Source: CAD feature listing. Evaluate the final solid. Frame: model axes, mm. Face numbers are marked on the shaded views. A direction names the side the tool comes from. Round coordinates to 2 decimals unless told otherwise and drop trailing zeros. Loops run counter-clockwise (first coordinate to the right, second up) from the corner with the lowest first, then second, coordinate; pieces in that order, holes last. Notation, with made-up numbers: M 5,41.5 L 49,41.5 A21 ccw 49,77.5 Z; hole C 70,87.5 d9. An arc over 180 degrees is marked long. Answer as CSV lines item,"result". Start each with the question number.
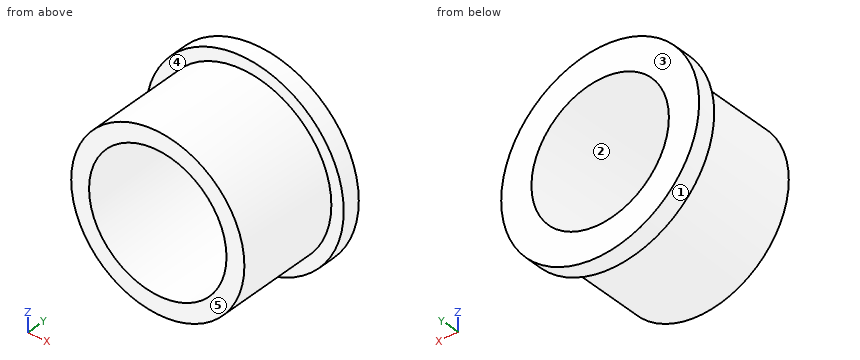
Autodesk Inventor part; units mm, degrees
ref_plane "YZ Plane" through (0, 0, 0) normal (1, 0, 0) x (0, 1, 0)
ref_plane "XZ Plane" through (0, 0, 0) normal (0, 1, 0) x (-1, 0, 0)
ref_plane "XY Plane" through (0, 0, 0) normal (0, 0, 1) x (1, 0, 0)
sketch "Sketch1" plane through (0, 0, 0) normal (0, 0, 1) x (1, 0, 0)
  line L0 (0, 0) -> (1.65, 0)
  line L1 (1.65, 0) -> (1.65, 3)
  line L2 (1.65, 3) -> (3.6, 3)
  line L3 (3.6, 3) -> (3.6, 3.65)
  line L4 (3.6, 3.65) -> (1.65, 3.65)
  line L5 (0, 0) -> (0, 3.65)
  line L6 (1.65, 3.65) -> (0, 3.65)
  dimension "d0" = 1.65
  dimension "d1" = 1.95
  dimension "d2" = 3
  dimension "d3" = 0.65
revolve "Revolution1" add sketch "Sketch1" angle 360 about axis through (0, 0, 0) along (0, 1, 0)
sketch "Sketch2" plane through (0, 0, 0) normal (1, 0, 0) x (0, 1, 0)
  line L0 (3, 1.65) -> (3, -1.65)
  line L1 (0, 1.65) -> (0, -1.65)
  line L2 (3.65, 3.6) -> (3.65, -3.6)
  line L3 (3, 3.6) -> (3, -3.6)
  line L4 (3, -1.65) -> (0, -1.65)
  line L5 (3, 1.65) -> (0, 1.65)
  line L6 (3, -3.15) -> (-0.75, -3.15)
  line L7 (-0.75, -3.15) -> (-0.75, -1.65)
  line L8 (-0.75, -1.65) -> (3, -1.65)
  line L9 (3, -1.65) -> (3, -3.15)
  line L10 (0, 0) -> (11.9884, 0)
  dimension "d5" = 3.75
  dimension "d6" = 1.5
  dimension "d12" = 3.15
sketch "Sketch3" plane through (0, 3.65, 0) normal (0, 1, 0) x (1, 0, 0)
  circle A0 centre (0, 0) radius 2.5
  dimension "d7" = 5
revolve "Revolution2" add sketch "Sketch2" angle 360 about axis through (0, 0, 0) along (0, 1, 0) contours L3 L6 L7 L8 L4
extrude "Extrusion1" cut sketch "Sketch3" against normal through all
properties part number "LED holder" material "ABS Plastic"
1) Access query for the marked faces 4 and 5. Directions: +Z, -Z, +X, -X, +Y, -Y. A direction counts if a zero-diameter tool reaches every point of the face in a straight line with its end or side. Return the directions, or none.
2) Section C-C, the plane y = 0.3. Return loops of the section in (x, z), and give its area (3 significant figures).
3) Mould query, pull axis Z, two halves, no side actions, for the marked faces 1, 2 and 3. Classes: pulls with the +Z half, pulls with the -Z half, needs draft (parallel to the pull), parting line crosses it, or undercut.
4) Ray query, line 1 along Z through (x, y) = (0, 0.4); line 2 along X through (y, z) = (1.6, 2.25). Return the intervals inside material, ascending.
5) Section B-B, the plane z = 0. Return loops of the section in (x, y), and give its area (4 significant figures).
6) Section A-A, the plane x = 0. Return loops of the section in (y, z).
Findings below:
1,face 4,"-Y"
1,face 5,"+Z, -Z, +X, -X, -Y"
2,outline,"C 0,0 d6.3; hole C 0,0 d5"
2,area,"11.5 mm²"
3,face 1,"parting line crosses it"
3,face 2,"undercut"
3,face 3,"needs draft"
4,line 1,"-3.15 to -2.5, 2.5 to 3.15"
4,line 2,"-2.2 to -1.09, 1.09 to 2.2"
5,outline,"M -3.6,3 L -3.15,3 L -3.15,-0.75 L -2.5,-0.75 L -2.5,3.65 L -3.6,3.65 Z; M 2.5,-0.75 L 3.15,-0.75 L 3.15,3 L 3.6,3 L 3.6,3.65 L 2.5,3.65 Z"
5,area,"6.305 mm²"
6,outline,"M -0.75,-3.15 L 3,-3.15 L 3,-3.6 L 3.65,-3.6 L 3.65,-2.5 L -0.75,-2.5 Z; M -0.75,2.5 L 3.65,2.5 L 3.65,3.6 L 3,3.6 L 3,3.15 L -0.75,3.15 Z"
